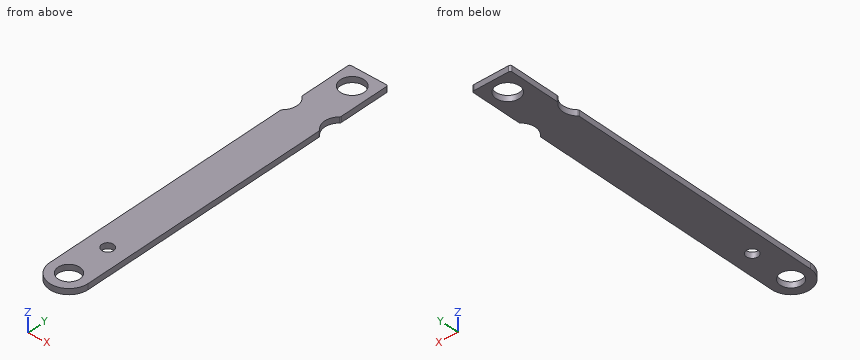
```python
from build123d import *

# Parameters (mm, degrees)
SKETCH_2_R      = 1.525
SKETCH_2_R_2    = 0.825
SKETCH_2_R_3    = 1.65
EXTRUDE_1_DEPTH = 0.8


with BuildPart() as part:
    # 草图2 → 凸台-拉伸1 (new body)
    with BuildSketch(Plane.XY):
        with BuildLine():
            Line((2.45, 46.401), (-2.45, 46.401))
            ThreePointArc((-2.45, 46.401), (-2.626776695, 46.327776695), (-2.7, 46.151))
            Line((-2.7, 46.151), (-2.7, 39.169281101))
            ThreePointArc((-2.7, 39.169281101), (-2.679315634, 39.069710321), (-2.620685279, 38.98661601))
            ThreePointArc((-2.620685279, 38.98661601), (-1.95, 37.442), (-2.620685279, 35.897383991))
            ThreePointArc((-2.620685279, 35.897383991), (-2.679315634, 35.814289679), (-2.7, 35.7147189))
            Line((-2.7, 35.7147189), (-2.7, 0))
            ThreePointArc((-2.7, 0), (0, -2.7), (2.7, 0))
            Line((2.7, 0), (2.7, 35.7147189))
            ThreePointArc((2.7, 35.7147189), (2.679315634, 35.814289679), (2.620685279, 35.897383991))
            ThreePointArc((2.620685279, 35.897383991), (1.95, 37.442), (2.620685279, 38.98661601))
            ThreePointArc((2.620685279, 38.98661601), (2.679315634, 39.069710321), (2.7, 39.169281101))
            Line((2.7, 39.169281101), (2.7, 46.151))
            ThreePointArc((2.7, 46.151), (2.626776695, 46.327776695), (2.45, 46.401))
        make_face()
        Circle(SKETCH_2_R, mode=Mode.SUBTRACT)
        with Locations((0, 6)):
            Circle(SKETCH_2_R_2, mode=Mode.SUBTRACT)
        with Locations((0, 43.851)):
            Circle(SKETCH_2_R_3, mode=Mode.SUBTRACT)
    extrude(amount=EXTRUDE_1_DEPTH)


solid = part.part
```
The listing builds one solid part. Answer for the finished solid, in the listing's coordinates (mm). Coordinates: 2 decimals unless noted, no trailing zeros. Order: outer loops, then holes, each group sorted by start corner. A loop starts at its lowest first (then second) coordinate and runs counter-clockwise, first axis right, second up. Notation, with made-up numbers: M 78,86.5 L 126,86.5 A9 cw 126,90.5 Z; hole C 48,79 d3. An arc over 180 degrees is marked long. Answer as a JSON object with one key per item and string values. Group by question number.
1. Section C-C on z = 0.45 is taken. Write down the section's boundary in (x, y) (3 decimals), then the cut area to 3 significant figures.
2. Section D-D on y = 43 is taken. Write down the section's boundary in (x, z), then the cut area to 3 significant figures.
3. Straight lines are drawn through the part: line 1 (Y direction, x = 0, z = 0.6) (3 decimals); line 2 (Y direction, x = -0.95, z = 0.25); line 3 (Y direction, x = -1.1, z = 0.75). For each, find the intervals that lie inside material, in ascending order.
4. Section A-A on y = 6 is taken. Write down the section's boundary in (x, z) (3 decimals).
5. Section B-B on x = 0 is taken. Write down the section's boundary in (y, z) (3 decimals).
6. A flat-ended cylindrical pin translates along its axis: P1, Ø3, axis at x = 0, y = 37.5, coming from the -Z side. Find the tip coordinate at first contact, or state that the pin passes through.
Values follow:
{
 "1": {"outline": "M -2.7,0 A2.7 ccw 2.7,0 L 2.7,35.715 A0.25 ccw 2.621,35.897 A2.114 cw 2.621,38.987 A0.25 ccw 2.7,39.169 L 2.7,46.151 A0.25 ccw 2.45,46.401 L -2.45,46.401 A0.25 ccw -2.7,46.151 L -2.7,39.169 A0.25 ccw -2.621,38.987 A2.114 cw -2.621,35.897 A0.25 ccw -2.7,35.715 Z; hole C 0,43.851 d3.3; hole C 0,0 d3.05; hole C 0,6 d1.65", "area": "241 mm2"},
 "2": {"outline": "M -2.7,0 L -1.41,0 L -1.41,0.8 L -2.7,0.8 Z; M 1.41,0 L 2.7,0 L 2.7,0.8 L 1.41,0.8 Z", "area": "2.06 mm2"},
 "3": {"line 1": "-2.7 to -1.525, 1.525 to 5.175, 6.825 to 42.201, 45.501 to 46.401", "line 2": "-2.53 to -1.19, 1.19 to 42.5, 45.2 to 46.4", "line 3": "-2.47 to -1.06, 1.06 to 42.62, 45.08 to 46.4"},
 "4": {"outline": "M -2.7,0 L -0.825,0 L -0.825,0.8 L -2.7,0.8 Z; M 0.825,0 L 2.7,0 L 2.7,0.8 L 0.825,0.8 Z"},
 "5": {"outline": "M -2.7,0 L -1.525,0 L -1.525,0.8 L -2.7,0.8 Z; M 1.525,0 L 5.175,0 L 5.175,0.8 L 1.525,0.8 Z; M 6.825,0 L 42.201,0 L 42.201,0.8 L 6.825,0.8 Z; M 45.501,0 L 46.401,0 L 46.401,0.8 L 45.501,0.8 Z"},
 "6": {"P1": "z = 0"}
}
